For this review, take the finished solid that the model builds, in its own axes (mm). Face numbers are marked on the shaded views. A direction names the side the tool comes from. Coordinates: 2 decimals unless noted, no trailing zeros. Write each loop counter-clockwise with the first axis right and the second up, starting at its lowest first coordinate (ties: lowest second). Pieces come first, ordered by that corner, then holes.
```python
from build123d import *

# Parameters (mm, degrees)
F0_W           = 140
F0_H           = 100
F1_DEPTH       = 5
F2_W           = 140
F2_H           = 100
F2_W_2         = 130
F2_H_2         = 90
F3_DEPTH       = 40
F5_D           = 3.3
F5_CBORE_D     = 6.5
F5_CBORE_DEPTH = 3
F7_D           = 10
F7_DEPTH       = 12
F7_TIP         = 3.0043030951
F9_D           = 10
F9_DEPTH       = 12
F9_TIP         = 3.0043030951
F10_W          = 5
F10_H          = 90
F11_DEPTH      = 5


with BuildPart() as f1:
    # F0 (on Top) → F1 (new body)
    with BuildSketch(Plane.XY):
        Rectangle(F0_W, F0_H)
    extrude(amount=F1_DEPTH)

    # F2 (on face) → F3 (join)
    with BuildSketch(Plane.XY.offset(5)):
        Rectangle(F2_W, F2_H)
        Rectangle(F2_W_2, F2_H_2, mode=Mode.SUBTRACT)
    extrude(amount=F3_DEPTH)

    # F5 (through all)
    with Locations(Plane(origin=(0, 0, 0), x_dir=(1, 0, 0), z_dir=(0, 0, -1))):
        with Locations((40.5, -4), (-14.5, -4)):
            CounterBoreHole(F5_D / 2, F5_CBORE_D / 2, F5_CBORE_DEPTH)

    # F7
    with Locations(Plane.YZ.offset(70)):
        with Locations((-40, 10)):
            Hole(F7_D / 2, depth=F7_DEPTH)
            with Locations((0, 0, -(F7_DEPTH + F7_TIP / 2))):  # 118° drill point
                Cone(0, F7_D / 2, F7_TIP, mode=Mode.SUBTRACT)

    # F9
    with Locations(Plane(origin=(-70, 0, 0), x_dir=(0, -1, 0), z_dir=(-1, 0, 0))):
        with Locations((-40, 10)):
            Hole(F9_D / 2, depth=F9_DEPTH)
            with Locations((0, 0, -(F9_DEPTH + F9_TIP / 2))):  # 118° drill point
                Cone(0, F9_D / 2, F9_TIP, mode=Mode.SUBTRACT)

    # F10 (on face) → F11 (cut)
    with BuildSketch(Plane.XY.offset(45)):
        with Locations((-67.5, 0)):
            Rectangle(F10_W, F10_H)
        with Locations((67.5, 0)):
            Rectangle(F10_W, F10_H)
    extrude(amount=-F11_DEPTH, mode=Mode.SUBTRACT)


solid = f1.part
```
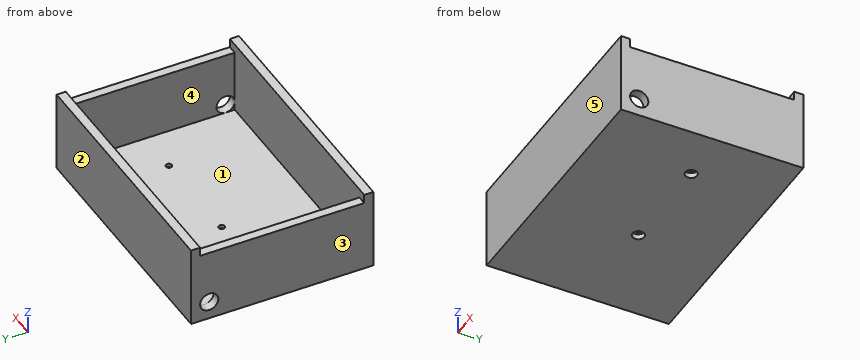
Q1. Add section A-A (y = 4). State the section outline as (x, z) points.
Ans:
outline: (-70, 0) - (-17.75, 0) - (-17.75, 3) - (-16.15, 3) - (-16.15, 5) - (-65, 5) - (-65, 40) - (-70, 40) - close; (-12.85, 3) - (-11.25, 3) - (-11.25, 0) - (37.25, 0) - (37.25, 3) - (38.85, 3) - (38.85, 5) - (-12.85, 5) - close; (42.15, 3) - (43.75, 3) - (43.75, 0) - (70, 0) - (70, 40) - (65, 40) - (65, 5) - (42.15, 5) - close
Q2. For probe 1 along X at (y, z) = (8, 10); probe 2 along Y at (x, z) = (37.5, 42); probe 3 along Z at (x, y) = (68, -40), list the stretches that pass through material, from the lowest coordinate up.
Ans:
probe 1: x = -70 to -65, 65 to 70
probe 2: y = -50 to -45, 45 to 50
probe 3: z = 0 to 5, 15 to 40
Q3. Tool access review of the marked faces 4 and 5: name each direction out of +Z, -Z, +X, -X, +Y, -Y from which nothing blocks a thin tool from reaching the whole face with its end or side.
Ans:
face 4: +Z
face 5: +Z, -Z, +X, -X, -Y
Q4. Add section C-C (z = 30). State the section outline as (x, y) points, then the cut area to 3 significant figures.
Ans:
outline: (-70, -50) - (70, -50) - (70, 50) - (-70, 50) - close; hole (-65, -45) - (65, -45) - (65, 45) - (-65, 45) - close
area: 2,300 mm2
Q5. Clearance check with flat-ended pins moving along their axes: pin 1 Ø4 at (x, y) = (-30.5, 1.5) entering from +Z; pin 2 Ø1.5 at (x, y) = (-67, -20) entering from +Z. State where each tip first meets the part, or that it passes through.
Ans:
pin 1: stops at z = 5
pin 2: stops at z = 40
Q6. Add section B-B (x = 40.5). State the section outline as (y, z) points, then the cut area to 3 significant figures.
Ans:
outline: (-50, 0) - (0.75, 0) - (0.75, 3) - (2.35, 3) - (2.35, 5) - (-45, 5) - (-45, 45) - (-50, 45) - close; (5.65, 3) - (7.25, 3) - (7.25, 0) - (50, 0) - (50, 45) - (45, 45) - (45, 5) - (5.65, 5) - close
area: 874 mm2
Q7. Add section D-D (y = -43). State the section outline as (x, z) points, then the cut area to 3 significant figures.
Ans:
outline: (-70, 0) - (70, 0) - (70, 6) - (65, 6) - (65, 5) - (-65, 5) - (-65, 40) - (-70, 40) - close; (65, 14) - (70, 14) - (70, 40) - (65, 40) - close
area: 1,010 mm2
Q8. Draft analysis for pull direction X (two halves, no side actions). For the marked faces 1, 2 and 3, state which applies: +X half, -X half, draft (parallel to the pull), parting line (faces both ways), or undercut.
Ans:
face 1: undercut
face 2: draft
face 3: -X half
